Geometry check sheet. Reference: the model listing, model coordinates, mm. A direction names the side the tool comes from. Round coordinates to 2 decimals unless told otherwise and drop trailing zeros. Loops run counter-clockwise (first coordinate to the right, second up) from the corner with the lowest first, then second, coordinate; pieces in that order, holes last. Notation, with made-up numbers: M 45,70 L 63,70 A30 ccw 63,93 Z; hole C 19,21 d8. An arc over 180 degrees is marked long. Use one line per item in the form item = value. Start each with the question number.
1. Cross-section at A-A (z = 3). Record the boundary of the cut face in (x, y), then the cut area to 3 significant figures.
2. Draft check along X on faces 1 (the cylindrical face through (120.83, 71.01, 17.5)), 2 (the cylindrical face through (59.25, 11.31, 6.26)), 3 (the flat face through (98, 49, 19.05)). Enter one of: pulls with the +X half, pulls with the -X half, needs draft (parallel to the pull), parting line crosses it, or undercut.
3. Material ranges on line 1 (Y direction, x = 96, z = 5); line 2 (Y direction, x = 40, z = 1); line 3 (Y direction, x = 123, z = 3), recorded low to high.
4. Set-up check for faces 4 (the cylindrical face through (72.205, 120.407, 17.504)), 5 (the cylindrical face through (74.518, 22.978, 7.888)): record each of +Z, -Z, +X, -X, +Y, -Y from which the full face is reachable in a straight line by a thin tool's end or side.
5. Go/stop test with flat-tipped pins: pin 1 (3.5 mm diameter, centred on x = 122.5, y = 73.5, fed in from +Z); pin 2 (4 mm diameter, centred on x = 87, z = 10, fed in from -Y); pin 3 (5 mm diameter, centred on x = 117.5, z = 17, fed in from -Y). Record where each tip stops, or that it passes through.
```python
from build123d import *

# Parameters (mm, degrees)
F0_R     = 63.453437
F0_R_2   = 3.689895
F0_R_3   = 25.381375
F1_DEPTH = 19.05
F0_R_4   = 1.586336
F2_DEPTH = 16
F3_R     = 6.35
F4_R     = 6.35


with BuildPart() as f1:
    # F0 (on Top) → F1 (new body)
    with BuildSketch(Plane.XY):
        with Locations((73.005051, 73.255326)):
            Circle(F0_R)
        with Locations((73.00505, 22.501889)):
            Circle(F0_R_2, mode=Mode.SUBTRACT)
        with Locations((22.251614, 73.255323)):
            Circle(F0_R_2, mode=Mode.SUBTRACT)
        with Locations((123.758487, 73.255323)):
            Circle(F0_R_2, mode=Mode.SUBTRACT)
        with Locations((73.00505, 124.008762)):
            Circle(F0_R_2, mode=Mode.SUBTRACT)
        with Locations((73.005051, 73.255326)):
            Circle(F0_R_3, mode=Mode.SUBTRACT)
    extrude(amount=F1_DEPTH)

    # F0 (on Top) → F2 (join)
    with BuildSketch(Plane.XY):
        with Locations((22.251614, 73.255323)):
            Circle(F0_R_2)
        with Locations((22.251614, 73.255323)):
            Circle(F0_R_4, mode=Mode.SUBTRACT)
        with Locations((73.00505, 22.501889)):
            Circle(F0_R_2)
        with Locations((73.00505, 22.501889)):
            Circle(F0_R_4, mode=Mode.SUBTRACT)
        with Locations((123.758487, 73.255323)):
            Circle(F0_R_2)
        with Locations((123.758487, 73.255323)):
            Circle(F0_R_4, mode=Mode.SUBTRACT)
        with Locations((73.00505, 124.008762)):
            Circle(F0_R_2)
        with Locations((73.00505, 124.008762)):
            Circle(F0_R_4, mode=Mode.SUBTRACT)
    extrude(amount=F2_DEPTH)

    # F3
    f3_edges = [f1.edges().sort_by_distance(p)[0] for p in [
        (9.551614, 73.255326, 19.05),
    ]]
    fillet(f3_edges, radius=F3_R)

    # F4
    f4_edges = [f1.edges().sort_by_distance(p)[0] for p in [
        (47.623676, 73.255326, 19.05),
    ]]
    fillet(f4_edges, radius=F4_R)


solid = f1.part
```
Reported:
q1.outline = C 73.01,73.26 d126.91; hole C 22.25,73.26 d3.17; hole C 73.01,73.26 d50.76; hole C 73.01,22.5 d3.17; hole C 73.01,124.01 d3.17; hole C 123.76,73.26 d3.17
q1.area = 10,600 mm²
q2.face_1 = undercut
q2.face_2 = parting line crosses it
q2.face_3 = needs draft
q3.line_1 = 14.12 to 62.51, 84 to 132.4
q3.line_2 = 19.06 to 127.45
q3.line_3 = 34.18 to 71.86, 74.65 to 112.33
q4.face_4 = +Z
q4.face_5 = +Z, -Z
q5.pin_1 = 16
q5.pin_2 = 10.95
q5.pin_3 = 27.01
